Can you work these out from the model? Positions are in its coordinate system, mm. A direction names the side the tool comes from. Give positions to 0.01 mm unless a question says otherwise; leave off trailing zeros. Write each loop counter-clockwise with the first axis right and the second up, starting at its lowest first coordinate (ties: lowest second). Pieces come first, ordered by that corner, then holes. Notation, with made-up numbers: M 45.5,75 L 98.5,75 A20 cw 98.5,96 Z; hole C -11,72 d5. An arc over 180 degrees is marked long. Use CSV: the item, a comma, the result in double quotes. Start each with the question number.
Autodesk Inventor part; units mm, degrees
ref_plane "YZ Plane" through (0, 0, 0) normal (1, 0, 0) x (0, 1, 0)
ref_plane "XZ Plane" through (0, 0, 0) normal (0, 1, 0) x (-1, 0, 0)
ref_plane "XY Plane" through (0, 0, 0) normal (0, 0, 1) x (1, 0, 0)
sketch "Sketch1" plane through (0, 0, 0) normal (0, 0, 1) x (1, 0, 0)
  line L0 (-75, 25) -> (75, 25)
  line L1 (75, 25) -> (75, -25)
  line L2 (75, -25) -> (-75, -25)
  line L3 (-75, -25) -> (-75, 25)
  line L4 (-75, 25) -> (75, -25) construction
  line L5 (75, 25) -> (-75, -25) construction
  line L6 (25, 25) -> (25, -25)
  line L7 (22.5, 25) -> (27.5, 25)
  line L8 (27.5, 25) -> (27.5, -25)
  line L9 (27.5, -25) -> (22.5, -25)
  line L10 (22.5, -25) -> (22.5, 25)
  line L11 (22.5, 25) -> (27.5, -25) construction
  line L12 (27.5, 25) -> (22.5, -25) construction
  line L13 (75, 25) -> (70, 25)
  line L14 (70, 25) -> (70, -25)
  line L15 (70, -25) -> (75, -25)
  line L16 (75, -25) -> (75, 25)
  point P0 (0, 0)
  point P1 (25, 0)
  point P2 (22.5, 25)
  point P3 (22.5, -25)
  point P4 (27.5, -25)
  point P5 (27.5, 25)
  dimension "d0" = 50
  dimension "d1" = 150
  dimension "d9" = 50
  dimension "d14" = 5
  dimension "d15" = 5
sketch "Sketch2" plane through (0, 0, 0) normal (1, 0, 0) x (0, 1, 0)
  line L0 (25, 0) -> (-25, 0)
  line L1 (25, 0) -> (-25, 0)
  line L2 (-25, 0) -> (-25, 70)
  line L3 (-25, 70) -> (25, 70)
  line L4 (25, 70) -> (25, 0)
  line L5 (-20, 70) -> (5.4779, 0)
  line L6 (25, 5) -> (-25, 5)
  line L7 (-20, 70) -> (-20, 0)
  point P0 (0, 0)
  point P1 (5.4779, 0)
  point P2 (3.6581, 5)
  dimension "d2" = 70
  dimension "d3" = 5
  dimension "d5" = 5
  dimension "d20" = 20
extrude "Extrusion1" add sketch "Sketch2" along normal blind 75 contours L0 L7 L6 L5 | L0 L2 L6 L7 | L6 L7 L5 | L6 L2 L3 L7
extrude "Extrusion2" add sketch "Sketch2" along normal blind 75 contours L0 L5 L6 L4
extrude "Extrusion3" add sketch "Sketch1" along normal blind 70 contours L0 L1 L2 L14
extrude "Extrusion4" add sketch "Sketch1" along normal blind 70 contours L0 L6 L2 L10 | L0 L8 L2 L6
mirror "Mirror1" about plane through (0, 0, 0) normal (1, 0, 0)
fillet "Fillet1" radius 2 9 edges at (-27.5, 25, 37.5) (-22.5, 25, 37.5) (22.5, 25, 37.5) (27.5, 25, 37.5) (70, 25, 37.5) (-70, 25, 37.5) (-48.75, 25, 5) (0, 25, 5) (48.75, 25, 5)
fillet "Fillet2" radius 2 10 edges at (-25, 25, 70) (-22.5, 1.5, 70) (-27.5, 1.5, 70) (25, 25, 70) (27.5, 1.5, 70) (22.5, 1.5, 70) (73.5, 25, 70) (70, 1.5, 70) (-73.5, 25, 70) (-70, 1.5, 70)
sketch "Sketch3" plane through (75, -25, 0) normal (0, -1, 0) x (1, 0, 0)
  line L0 (0, 0) -> (-150, 0)
  line L1 (0, 70) -> (0, 0)
  line L2 (-150, 70) -> (0, 70)
  line L3 (-150, 70) -> (-150, 0)
  line L4 (-145, 5) -> (-5, 5)
  line L5 (-5, 5) -> (-5, 65)
  line L6 (-5, 65) -> (-145, 65)
  line L7 (-145, 65) -> (-145, 5)
  circle A0 centre (-5, 5) radius 2.7
  circle A1 centre (-145, 5) radius 2.75
  point P0 (-75, 0)
  dimension "d35" = 5
  dimension "d36" = 5.4
  dimension "d37" = 5.5
extrude "Extrusion5" cut sketch "Sketch3" against normal blind 10 contours L7 A1 L4 | L4 A1 L7 | A0 L5 L4 | L4 L5 A0
fillet "Fillet3" radius 1 2 edges at (67.3, -25, 5) (-72.75, -25, 5)
ref_plane "Work Plane2" through (75, -25, 5) normal (0, 0, -1) x (-1, 0, 0)
fillet "Fillet4" radius 1 1 edges at (-72.75, -15, 5)
fillet "Fillet5" radius 1 1 edges at (67.3, -15, 5)
sketch "Sketch4" plane through (75, 0, 0) normal (1, 0, 0) x (0, 0, -1)
  circle A0 centre (-62, -20) radius 1.875
  point P0 (0, 0)
  dimension "d44" = 3.75
extrude "Extrusion6" cut sketch "Sketch4" against normal blind 10
sketch "Sketch6" plane through (-75, -25, 0) normal (-1, 0, 0) x (0, 0, 1)
  circle A0 centre (41.25, 42.644) radius 1.95
  circle A1 centre (24.5833, 42.644) radius 1.95
  point P0 (0, 25)
  dimension "d52" = 3.9
  dimension "d53" = 3.9
extrude "Extrusion7" cut sketch "Sketch6" against normal blind 5
equation "\"d9\" = 0.333333 * d1"
equation "\"d5\" = d3"
equation "\"d10\" = 0.5 * d1"
equation "\"d12\" = 0.5 * d1"
equation "\"d16\" = d2"
equation "\"d18\" = d2"
properties part number "rubbish-container-group2" material "ABS Plastic"
(1) I want a section at A-A (z = 41.25). Write out the boundary of the cut face in (x, y), and give its area (3 significant figures).
(2) I want a section at B-B (x = -57). Write out the boundary of the cut face in (y, z), and give its area (3 significant figures).
(3) I want a section at D-D (z = 62). Write out the boundary of the cut face in (x, y) (3 decimals), and give its area (3 significant figures).
(4) Will these pins go through, and if not, where does the flat tip stop? pin 1 Ø10 at (x, z) = (11.5, 26) entering from +Y; pin 2 Ø3 at (y, z) = (17.644, 41.25) entering from -X; pin 3 Ø1.1 at (y, z) = (-20, 61.5) entering from +X; pin 4 Ø4 at (y, z) = (17.5, 39.5) entering from -X.
(5) Please list where these lines run through material, in increasing order: L1, parallel to X at y = -1, z = 57; L2, parallel to Y at x = -72.9, z = 41.25; L3, parallel to Z at x = 36, y = 11.5. Write a range as [from, to].
(6) I want a section at C-C (y = -7). Write out the boundary of the cut face in (x, z), and give its area (3 significant figures).
(7) Thinking about a two-plate mould opening in Z: for faces 4 (the face through (69.415, -20.056, 2.364)), 5 (the face through (48, 13, 5)), 6 (the face through (-1, 0, 0)), 7 (the face through (70, 7, 43)), which applies, released by +Z, released by -Z, zero draft, split by the parting line, or undercut?
(8) Which directions (+Z, -Z, +X, -X, +Y, -Y) give clear straight access to the entire face, cutting with the end or side of a thin tool? Please do faces 1 (the face through (-48.424, -8.005, 37.045)), 2 (the face through (-72.535, 16.897, 43.051)), 3 (the face through (65, -20, 62)).
Geometry results:
1,outline,"M -75,-25 L 75,-25 L 75,25 L 72,25 A2 ccw 70,23 L 70,-9.54 L 27.5,-9.54 L 27.5,23 A2 ccw 25.5,25 L 24.5,25 A2 ccw 22.5,23 L 22.5,-9.54 L -22.5,-9.54 L -22.5,23 A2 ccw -24.5,25 L -25.5,25 A2 ccw -27.5,23 L -27.5,-9.54 L -70,-9.54 L -70,15.69 L -75,15.69 Z; M -75,19.59 L -70,19.59 L -70,23 A2 ccw -72,25 L -75,25 Z"
1,area,"2,990 mm2"
2,outline,"M -25,0 L 25,0 L 25,3 A2 ccw 23,5 L 3.66,5 L -20,70 L -25,70 Z"
2,area,"1,340 mm2"
3,outline,"M -75,-25 L 75,-25 L 75,-21.875 L 65,-21.875 L 65,-18.125 L 75,-18.125 L 75,25 L 72,25 A2 ccw 70,23 L 70,-17.088 L 27.5,-17.088 L 27.5,23 A2 ccw 25.5,25 L 24.5,25 A2 ccw 22.5,23 L 22.5,-17.088 L -22.5,-17.088 L -22.5,23 A2 ccw -24.5,25 L -25.5,25 A2 ccw -27.5,23 L -27.5,-17.088 L -70,-17.088 L -70,23 A2 ccw -72,25 L -75,25 Z"
3,area,"1,990 mm2"
4,pin 1,"stops at y = -2.17"
4,pin 2,"stops at x = -27.5"
4,pin 3,"stops at x = 65"
4,pin 4,"stops at x = -75"
5,L1,"x = [-75, -70], [-27.5, -22.5], [22.5, 27.5], [70, 75]"
5,L2,"y = [-25, 15.69], [19.59, 25]"
5,L3,"z = [0, 5]"
6,outline,"M -75,0 L 75,0 L 75,70 L 72,70 A2 ccw 70,68 L 70,34.28 L 27.5,34.28 L 27.5,68 A2 ccw 25.5,70 L 24.5,70 A2 ccw 22.5,68 L 22.5,34.28 L -22.5,34.28 L -22.5,68 A2 ccw -24.5,70 L -25.5,70 A2 ccw -27.5,68 L -27.5,34.28 L -70,34.28 L -70,68 A2 ccw -72,70 L -75,70 Z"
6,area,"5,850 mm2"
7,face 4,"undercut"
7,face 5,"released by +Z"
7,face 6,"released by -Z"
7,face 7,"zero draft"
8,face 1,"+Z, +Y"
8,face 2,"-X"
8,face 3,"+X"
